Source: CAD feature listing. Evaluate the final solid. Frame: model axes, mm. A direction names the side the tool comes from. Round coordinates to 2 decimals unless told otherwise and drop trailing zeros. Order: outer loops, then holes, each group sorted by start corner. A loop starts at its lowest first (then second) coordinate and runs counter-clockwise, first axis right, second up. Notation, with made-up numbers: (-35, 54) -> (7, 54) arc R11 ccw to (7, 62) -> close; hole circle Ø10 at (-37, 89). An arc over 180 degrees is marked (long way). Write item = value, one per line. Start each with the question number.
(1) Cut plane A-A on x = -19. Return the cut outline in (y, z), then the cut area to 3 significant figures.
(2) Ray query, line 1 (Z direction, x = -19, y = 1.3); line 2 (Z direction, x = -25.5, y = 10.75); line 3 (X direction, y = 13.5, z = -6). Return the intervals inside material, ascending.
(3) Reachability of faces 4 (the face through (7, 2, -25)), 5 (the face through (-19, 2, -52)), 6 (the face through (-19, 20, -25)), 7 (the face through (-19, 2, 2)) from +Z, -Z, +X, -X, +Y, -Y: full face, straight path, thin tool, end or side. Return the list, or none.
(4) Cut plane B-B on z = 4. Return the cut outline in (x, y), then the cut area to 3 significant figures.
(5) Cut plane C-C on z = -3. Return the cut outline in (x, y), then the cut area to 3 significant figures.
(6) Draft query along Z for faces 1 (the face through (-19, 1, -57)), 2 (the face through (0, 11, -25)), 3 (the face through (-20.2, 1, -54.9)). Return one class per face: released by +Z, released by -Z, zero draft, split by the parting line, or undercut.
(7) Cut plane D-D on y = 11. Return the cut outline in (x, z), then the cut area to 3 significant figures.
(8) Contact query for flat-ended pins moving along their axis: pin 1 Ø1.5 at (x, y) = (-26, 3) entering from +Z; pin 2 Ø12 at (x, z) = (4.5, -13.5) entering from +Y; pin 3 Ø2 at (x, z) = (-18, 3.5) entering from +Y; pin 4 Ø1.5 at (y, z) = (3, -34) entering from +X. Output: stop coordinate, or through.
Autodesk Inventor part; units mm, degrees
ref_plane "Work Plane1" through (-38, 20, -25) normal (0, 0, 1) x (1, 0, 0)
ref_plane "YZ Plane" through (0, 0, 0) normal (1, 0, 0) x (0, 1, 0)
ref_plane "XZ Plane" through (0, 0, 0) normal (0, 1, 0) x (-1, 0, 0)
sketch "Sketch1" plane through (0, 0, 0) normal (0, 1, 0) x (-1, 0, 0)
  line L0 (0, 0) -> (38, 0)
  line L1 (38, 0) -> (38, -50)
  line L2 (38, -50) -> (0, -50)
  line L3 (0, -50) -> (0, 0)
  dimension "d0" = 38
  dimension "d1" = 50
extrude "Extrusion1" add sketch "Sketch1" along normal blind 20
sketch "Sketch2" plane through (0, 0, 0) normal (0, -1, 0) x (1, 0, 0)
  line L0 (0, 0) -> (0, -50)
  line L1 (0, 0) -> (15, 0)
  line L2 (15, 0) -> (15, -50)
  line L3 (15, -50) -> (0, -50)
  line L4 (0, -50) -> (0, 0)
  dimension "d4" = 15
  dimension "d5" = 50
extrude "Extrusion2" add sketch "Sketch2" against normal blind 2
sketch "Sketch3" plane through (0, 0, 0) normal (0, -1, 0) x (1, 0, 0)
  line L0 (-38, 0) -> (0, 0)
  line L1 (-19, 0) -> (-19, 7)
  line L2 (-19, 0) -> (-19, 4)
  line L3 (-19, 0) -> (-10.5, 0)
  line L4 (-19, 0) -> (-27.5, 0)
  circle A0 centre (-19, 4) radius 1.5
  circle A1 centre (-19, 4) radius 3
  line L5 (-10.5, 0) -> (-17.5, 6.5981)
  line L6 (-27.5, 0) -> (-20.5, 6.5981)
  dimension "d8" = 7
  dimension "d9" = 4
  dimension "d10" = 8.5
  dimension "d11" = 8.5
  dimension "d12" = 3
  dimension "d13" = 6.5981
  dimension "d14" = 6.5981
extrude "Extrusion3" add sketch "Sketch3" against normal blind 2 contours L6 A1 L1 L0 | L1 A1 L5 L0 | L6 A1 L1 A0 | L1 A0 A1 L5
ref_plane "Work Plane1" through (-38, 20, -25) normal (0, 0, 1) x (1, 0, 0)
mirror "Mirror1" about plane through (-38, 20, -25) normal (0, 0, 1) of "Extrusion3"
properties part number "25W_1224_5V"
Evaluation:
q1.outline = (0, -57) -> (2, -57) -> (2, -55.5) -> (0, -55.5) -> close; (0, -52.5) -> (2, -52.5) -> (2, -50) -> (20, -50) -> (20, 0) -> (2, 0) -> (2, 2.5) -> (0, 2.5) -> close; (0, 5.5) -> (2, 5.5) -> (2, 7) -> (0, 7) -> close
q1.area = 1,020 mm^2
q2.line_1 = -57 to -55.5, -52.5 to 2.5, 5.5 to 7
q2.line_2 = -50 to 0
q2.line_3 = -38 to 0
q3.face_4 = +Z, -Z, +X, +Y
q3.face_5 = -Z, +X, -X, +Y
q3.face_6 = +Z, -Z, +X, -X, +Y
q3.face_7 = +Z, +X, -X, +Y
q4.outline = (-23.26, 0) -> (-20.5, 0) -> (-20.5, 2) -> (-23.26, 2) -> close; (-17.5, 0) -> (-14.74, 0) -> (-14.74, 2) -> (-17.5, 2) -> close
q4.area = 11.0 mm^2
q5.outline = (-38, 0) -> (15, 0) -> (15, 2) -> (0, 2) -> (0, 20) -> (-38, 20) -> close
q5.area = 790 mm^2
q6.face_1 = released by -Z
q6.face_2 = zero draft
q6.face_3 = undercut
q7.outline = (-38, -50) -> (0, -50) -> (0, 0) -> (-38, 0) -> close
q7.area = 1,900 mm^2
q8.pin_1 = 0
q8.pin_2 = 20
q8.pin_3 = 2
q8.pin_4 = 0
